For this review, take the finished solid that the model builds, in its own axes (mm). Face numbers are marked on the shaded views. A direction names the side the tool comes from. Give positions to 0.01 mm unless a question says otherwise; leave off trailing zeros. Order: outer loops, then holes, each group sorted by start corner. A loop starts at its lowest first (then second) coordinate and runs counter-clockwise, first axis right, second up.
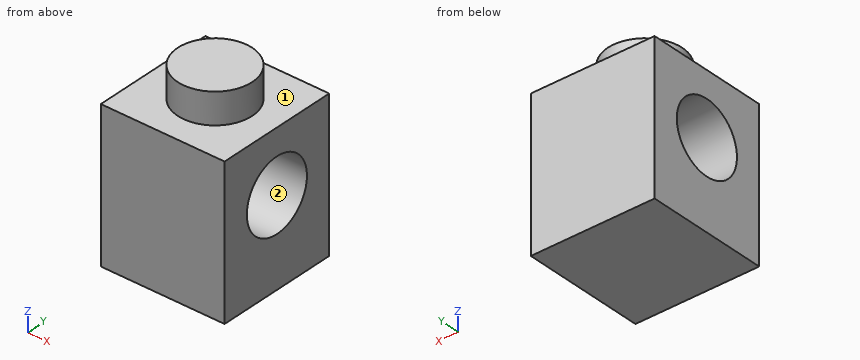
from build123d import *

# Parameters (mm, degrees)
F0_W     = 8
F0_H     = 8
F1_DEPTH = 9.6
F2_R     = 2.3
F3_DEPTH = 25
F4_R     = 2.4
F5_DEPTH = 2


with BuildPart() as f1:
    # F0 (on Top) → F1 (new body)
    with BuildSketch(Plane.XY):
        with Locations((-38.088854, 27.291242)):
            Rectangle(F0_W, F0_H)
    extrude(amount=F1_DEPTH)

    # F2 (on face) → F3 (cut)
    with BuildSketch(Plane.YZ.offset(-34.088854)):
        with Locations((27.291242, 5.6)):
            Circle(F2_R)
    extrude(amount=-F3_DEPTH, mode=Mode.SUBTRACT)

    # F4 (on face) → F5 (join)
    with BuildSketch(Plane.XY.offset(9.6)):
        with Locations((-38.088854, 27.291242)):
            Circle(F4_R)
    extrude(amount=F5_DEPTH)


solid = f1.part
1) Tool access review of the marked faces 1 and 2: name each direction out of +Z, -Z, +X, -X, +Y, -Y from which nothing blocks a thin tool from reaching the whole face with its end or side.
Answer sheet:
face 1: +Z
face 2: +X, -X
2) We need section A-A on z = 5.6. Give the boundary of the cut face in (x, y), then the cut area to 3 significant figures.
Answer sheet:
outline: (-42.09, 23.29) - (-34.09, 23.29) - (-34.09, 24.99) - (-42.09, 24.99) - close; (-42.09, 29.59) - (-34.09, 29.59) - (-34.09, 31.29) - (-42.09, 31.29) - close
area: 27.2 mm2
3) To check wall thickness, follow line 1 (Z direction, x = -36.5, y = 26.5); line 2 (Y direction, x = -36, z = 3.75); line 3 (Z direction, x = -39.25, y = 25.75). State the ranges of each line that lie inside material, in increasing order.
Answer sheet:
line 1: z = 0 to 3.44, 7.76 to 11.6
line 2: y = 23.29 to 25.92, 28.66 to 31.29
line 3: z = 0 to 3.89, 7.31 to 11.6
4) We need section D-D on y = 30. Give the boundary of the cut face in (x, z), then the cut area to 3 significant figures.
Answer sheet:
outline: (-42.09, 0) - (-34.09, 0) - (-34.09, 9.6) - (-42.09, 9.6) - close
area: 76.8 mm2
5) We need section B-B on x = -39.25. Give the boundary of the cut face in (y, z).
Answer sheet:
outline: (23.29, 0) - (31.29, 0) - (31.29, 9.6) - (29.39, 9.6) - (29.39, 11.6) - (25.19, 11.6) - (25.19, 9.6) - (23.29, 9.6) - close; hole circle Ø4.6 at (27.29, 5.6)
6) We need section C-C on y = 28. Give the boundary of the cut face in (x, z).
Answer sheet:
outline: (-42.09, 0) - (-34.09, 0) - (-34.09, 3.41) - (-42.09, 3.41) - close; (-42.09, 7.79) - (-34.09, 7.79) - (-34.09, 9.6) - (-35.8, 9.6) - (-35.8, 11.6) - (-40.38, 11.6) - (-40.38, 9.6) - (-42.09, 9.6) - close
